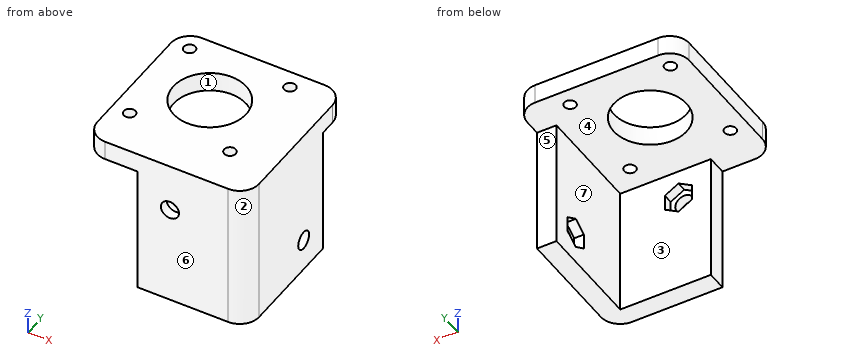
from build123d import *

# Parameters (mm, degrees)
SKETCH1_W              = 50
SKETCH1_H              = 50
BOSS_EXTRUDE1_DEPTH    = 6
BOSS_EXTRUDE2_DEPTH    = 40
F_3_6MM_DOWEL_HOLE1_D  = 3.6
F_22_5MM_DOWEL_HOLE1_D = 22.5
F_5_6MM_DOWEL_HOLE1_D  = 5.6
F_5_6MM_DOWEL_HOLE2_D  = 5.6
CUT_EXTRUDE1_DEPTH     = 3
CUT_EXTRUDE2_DEPTH     = 3
FILLET1_R              = 6


with BuildPart() as part:
    # Sketch1 → Boss-Extrude1 (new body)
    with BuildSketch(Plane.XY):
        with Locations((-25, 25)):
            Rectangle(SKETCH1_W, SKETCH1_H)
    extrude(amount=-BOSS_EXTRUDE1_DEPTH)

    # Sketch2 → Boss-Extrude2 (add)
    with BuildSketch(Plane(origin=(0, 0, -6), x_dir=(-1, 0, 0), z_dir=(0, 0, -1))):
        Polygon((0, 39), (6, 39), (6, 6), (34, 6), (34, 0), (6, 0), (0, 0), align=None)
    extrude(amount=BOSS_EXTRUDE2_DEPTH)

    # Ø3.6mm Dowel Hole1 (through all)
    with Locations(Plane.XY):
        with Locations((-44.5, 44.5), (-13.5, 44.5), (-13.5, 13.5), (-44.5, 13.5)):
            Hole(F_3_6MM_DOWEL_HOLE1_D / 2)

    # Ø22.5mm Dowel Hole1 (through all)
    with Locations(Plane.XY):
        with Locations((-29, 29)):
            Hole(F_22_5MM_DOWEL_HOLE1_D / 2)

    # Ø5.6mm Dowel Hole1 (through all)
    with Locations(Plane(origin=(0, 29, -36), x_dir=(0, 0, 1), z_dir=(1, 0, 0))):
        with Locations((0, 0)):
            Hole(F_5_6MM_DOWEL_HOLE1_D / 2)

    # Ø5.6mm Dowel Hole2 (through all)
    with Locations(Plane(origin=(0, 0, 0), x_dir=(-1, 0, 0), z_dir=(0, -1, 0))):
        with Locations((24, 15)):
            Hole(F_5_6MM_DOWEL_HOLE2_D / 2)

    # Sketch12 → Cut-Extrude1 (cut)
    with BuildSketch(Plane(origin=(0, 6, 0), x_dir=(1, 0, 0), z_dir=(0, 1, 0))):
        Polygon((-28.2, 12.575128869), (-24, 10.150257739), (-19.8, 12.575128869), (-19.8, 17.424871131), (-24, 19.849742261), (-28.2, 17.424871131), align=None)
    extrude(amount=-CUT_EXTRUDE1_DEPTH, mode=Mode.SUBTRACT)

    # Sketch13 → Cut-Extrude2 (cut)
    with BuildSketch(Plane.ZY.offset(6)):
        Polygon((-40.849742261, 29), (-38.424871131, 24.8), (-33.575128869, 24.8), (-31.150257739, 29), (-33.575128869, 33.2), (-38.424871131, 33.2), align=None)
    extrude(amount=-CUT_EXTRUDE2_DEPTH, mode=Mode.SUBTRACT)

    # Fillet1
    fillet1_edges = [part.edges().sort_by_distance(p)[0] for p in [
        (-50, 50, -3),
        (0, 50, -3),
        (0, 0, -23),
        (-50, 0, -3),
    ]]
    fillet(fillet1_edges, radius=FILLET1_R)


solid = part.part
Can you work these out from the model? Positions are in its coordinate system, mm. Face numbers are marked on the shaded views. A direction names the side the tool comes from. Round coordinates to 2 decimals unless told otherwise and drop trailing zeros. Order: outer loops, then holes, each group sorted by start corner. A loop starts at its lowest first (then second) coordinate and runs counter-clockwise, first axis right, second up. Notation, with made-up numbers: M -10.5,-5 L 10.5,-5 A28 ccw 10.5,23 Z; hole C -37.75,88 d5. An arc over 180 degrees is marked long. Use a Markdown table: item, result.
1) Imagine slicing it at B-B (x = -13.5). List the corners of the cut face in (y, z) for me, then the cut area to 3 significant figures.
Geometry says:
| item | result |
|---|---|
| outline | M 0,-46 L 6,-46 L 6,-6 L 11.7,-6 L 11.7,0 L 0,0 Z; M 15.3,-6 L 42.7,-6 L 42.7,0 L 15.3,0 Z; M 46.3,-6 L 50,-6 L 50,0 L 46.3,0 Z |
| area | 497 mm² |
2) If we mould it in two halves opening along Y, with no side actions, what happens to the marked faces 1, 2, 3 and 4? For each: +Y half, -Y half, draft (parallel to the pull), parting line (faces both ways), or undercut.
Geometry says:
| item | result |
|---|---|
| face 1 | undercut |
| face 2 | -Y half |
| face 3 | +Y half |
| face 4 | draft |
3) I'm going to push flat-ended pins straight in: P1, Ø4, axis at x = -13.5, y = 44.5, coming from the +Z side; P2, Ø2.5, axis at y = 4.5, z = -16, coming from the +X side; P3, Ø8, axis at x = -33, z = -13.5, coming from the +Y side; P4, Ø10, axis at x = -17.5, y = 30.5, coming from the -Z side. Where does each tip first touch, or does it pass through?
Geometry says:
| item | result |
|---|---|
| P1 | stops at z = 0 |
| P2 | stops at x = -0.01 |
| P3 | stops at y = 6 |
| P4 | stops at z = -6 |
4) On a 3-axis mill with a long thin cutter (end or side, diameter ignored), from which of +Z, -Z, +X, -X, +Y, -Y can I reach the whole of each face in a straight line? I mean the marked faces 5, 6 and 7. Say none if no direction works.
Geometry says:
| item | result |
|---|---|
| face 5 | -Z, +X, -X, +Y |
| face 6 | +Z, -Z, +X, -X, -Y |
| face 7 | -Z, -X, +Y |
5) Imagine slicing it at A-A (z = -15). List the corners of the cut face in (x, y) for me.
Geometry says:
| item | result |
|---|---|
| outline | M -34,0 L -26.8,0 L -26.8,3 L -28.2,3 L -28.2,6 L -34,6 Z; M -21.2,0 L -6,0 A6 ccw 0,6 L 0,39 L -6,39 L -6,6 L -19.8,6 L -19.8,3 L -21.2,3 Z |
6) Imagine slicing it at D-D (z = -27). List the corners of the cut face in (x, y) for me, then the cut area to 3 significant figures.
Geometry says:
| item | result |
|---|---|
| outline | M -34,0 L -6,0 A6 ccw 0,6 L 0,39 L -6,39 L -6,6 L -34,6 Z |
| area | 394 mm² |
7) Imagine slicing it at C-C (y = 13.5). List the corners of the cut face in (x, z) for me, then the cut area to 3 significant figures.
Geometry says:
| item | result |
|---|---|
| outline | M -50,-6 L -46.3,-6 L -46.3,0 L -50,0 Z; M -42.7,-6 L -15.3,-6 L -15.3,0 L -42.7,0 Z; M -11.7,-6 L -6,-6 L -6,-46 L 0,-46 L 0,0 L -11.7,0 Z |
| area | 497 mm² |
8) If I drill on line 1 along Y through (x, z) = (-13.5, -3.25); line 2 along X through (y, z) = (44, -2); line 3 along Y through (x, z) = (-44, -2), over which ranges is the centre line in solid material (lowest first)?
Geometry says:
| item | result |
|---|---|
| line 1 | y = 0 to 11.7, 15.3 to 42.7, 46.3 to 50 |
| line 2 | x = -50 to -46.23, -42.77 to -15.23, -11.77 to 0 |
| line 3 | y = 0 to 11.77, 15.23 to 42.77, 46.23 to 50 |
